from build123d import *

# Parameters (mm, degrees)
SKETCH_1_R          = 2.5
EXTRUDE_1_DEPTH     = 10
CUT_EXTRUDE_1_DEPTH = 42.533119315


with BuildPart() as part:
    # 草图1 → 凸台-拉伸1 (new, symmetric)
    with BuildSketch(Plane.XY):
        with BuildLine():
            Line((0, 10), (0, -10))
            Line((0, -10), (-30.8112495, -4.933748499))
            ThreePointArc((-30.8112495, -4.933748499), (-35, 0), (-30.8112495, 4.933748499))
            Line((-30.8112495, 4.933748499), (0, 10))
        make_face()
        with Locations((-30, 0)):
            Circle(SKETCH_1_R, mode=Mode.SUBTRACT)
    extrude(amount=EXTRUDE_1_DEPTH, both=True)

    # 草图2 → 切除-拉伸1 (cut, through all)
    with BuildSketch(Plane.XY.offset(10)):
        with BuildLine():
            Line((-25.960774055, -3.704449068), (-2, -7.644286286))
            Line((-2, -7.644286286), (-2, 7.644286286))
            Line((-2, 7.644286286), (-25.960774055, 3.704449068))
            ThreePointArc((-25.960774055, 3.704449068), (-24.519280236, 0), (-25.960774055, -3.704449068))
        make_face()
    extrude(amount=-CUT_EXTRUDE_1_DEPTH, mode=Mode.SUBTRACT)


solid = part.part
Source: CAD feature listing. Evaluate the final solid. Frame: model axes, mm. A direction names the side the tool comes from. Round coordinates to 2 decimals unless told otherwise and drop trailing zeros. Write each loop counter-clockwise with the first axis right and the second up, starting at its lowest first coordinate (ties: lowest second). Pieces come first, ordered by that corner, then holes. Notation, with made-up numbers: M 34,-14.5 L 91,-14.5 A23 cw 91,20.5 Z; hole C 3,77.5 d10. An arc over 180 degrees is marked long. One line per item, written item: value. Start each with the question number.
Item 1: Section query C-C (y = 5.75). Return the cut outline in (x, z), plus the area to 3 significant figures.
Item 2: Section query A-A (z = 5.5). Return the cut outline in (x, y), plus the area to 3 significant figures.
Item 3: Pin query (flat end, axial travel): pin 1 (1.5 mm diameter, centred on y = 1.5, z = 6.5, fed in from -X); pin 2 (3 mm diameter, centred on x = -19, z = -6.5, fed in from -Y); pin 3 (5 mm diameter, centred on y = 3, z = 1.5, fed in from -X); pin 4 (4.5 mm diameter, centred on x = -30, y = 0, fed in from +Z). Return the tip coordinate at first contact, or that it passes through.
Item 4: Section query D-D (x = -21.5). Return the cut outline in (y, z).
Item 5: Ray query, L1, parallel to X at y = -1.25, z = 2.75; L2, parallel to X at y = -1.75, z = 9.25; L3, parallel to X at y = 3, z = -5.25. Return the intervals inside material, ascending. Write a range as from..to.
Item 6: Mould query, pull axis X, two halves, no side actions, for faces 1 (the flat face through (-18.7, 5.2, -10)), 2 (the flat face through (-15.2, -7.5, 0.1)), 3 (the cylindrical face through (-24.52, 0.06, 0.14)), 4 (the cylindrical face through (-32.5, 0.1, -0.1)). Classes: pulls with the +X half, pulls with the -X half, needs draft (parallel to the pull), parting line crosses it, or undercut.
Item 7: Set-up query: faces 5 (the flat face through (-2, 0, 0)), 6 (the flat face through (-18.7, 5.2, 10)). Return all of +Z, -Z, +X, -X, +Y, -Y with unobstructed straight access to the full face (end or side cutting, diameter ignored); none if empty.
Item 8: Section query B-B (y = 0). Return the cut outline in (x, z).
Result set:
1. outline: M -25.85,-10 L -13.52,-10 L -13.52,10 L -25.85,10 Z; M -2,-10 L 0,-10 L 0,10 L -2,10 Z
1. area: 287 mm²
2. outline: M -30.81,-4.93 L 0,-10 L 0,10 L -30.81,4.93 A5 ccw Z; hole C -30,0 d5; hole M -25.96,-3.7 L -2,-7.64 L -2,7.64 L -25.96,3.7 A5.48 cw Z
2. area: 207 mm²
3. pin 1: stops at x = -34.94
3. pin 2: stops at y = -7.12
3. pin 3: stops at x = -34.97
3. pin 4: passes through
4. outline: M -6.46,-10 L -4.44,-10 L -4.44,10 L -6.46,10 Z; M 4.44,-10 L 6.46,-10 L 6.46,10 L 4.44,10 Z
5. L1: x = -34.84..-32.17, -27.83..-24.66, -2..0
5. L2: x = -34.68..-31.79, -28.21..-24.81, -2..0
5. L3: x = -34..-25.41, -2..0
6. face 1: needs draft
6. face 2: pulls with the -X half
6. face 3: undercut
6. face 4: undercut
7. face 5: +Z, -Z
7. face 6: +Z, +X, -X, +Y, -Y
8. outline: M -35,-10 L -32.5,-10 L -32.5,10 L -35,10 Z; M -27.5,-10 L -24.52,-10 L -24.52,10 L -27.5,10 Z; M -2,-10 L 0,-10 L 0,10 L -2,10 Z
